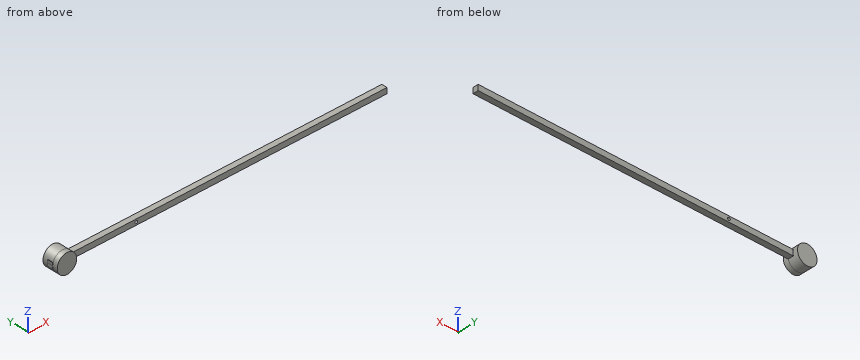
from build123d import *

# Parameters (mm, degrees)
F1_DEPTH      = 10
F3_DEPTH      = 8.75
F3_DEPTH_BACK = 18.75


with BuildPart() as f1:
    # F0 (on Front) → F1 (new body)
    with BuildSketch(Plane.XZ):
        with BuildLine():
            Line((-150, -5), (300, -5))
            Line((300, -5), (300, 5))
            Line((300, 5), (-150, 5))
            ThreePointArc((-150, 5), (-146.464466, 3.535534), (-145, 0))
            ThreePointArc((-145, 0), (-146.464466, -3.535534), (-150, -5))
        make_face()
        with BuildLine():
            Line((-300, -5), (-150, -5))
            ThreePointArc((-150, -5), (-153.535534, -3.535534), (-155, 0))
            Line((-155, 0), (-300, 0))
            Line((-300, 0), (-300, -5))
        make_face()
        with BuildLine():
            Line((-300, 0), (-155, 0))
            ThreePointArc((-155, 0), (-153.535534, 3.535534), (-150, 5))
            Line((-150, 5), (-300, 5))
            Line((-300, 5), (-300, 0))
        make_face()
        with BuildLine():
            ThreePointArc((-155, 0), (-153.535534, -3.535534), (-150, -5))
            ThreePointArc((-150, -5), (-146.464466, -3.535534), (-145, 0))
            ThreePointArc((-145, 0), (-146.464466, 3.535534), (-150, 5))
            ThreePointArc((-150, 5), (-153.535534, 3.535534), (-155, 0))
        make_face()
        with BuildLine():
            ThreePointArc((-147.5, 0), (-150, -2.5), (-152.5, 0))
            ThreePointArc((-152.5, 0), (-150, 2.5), (-147.5, 0))
        make_face(mode=Mode.SUBTRACT)
    extrude(amount=F1_DEPTH)

    # F2 (on face) → F3 (join, two sides)
    with BuildSketch(Plane.XZ.offset(10)) as f3_sk:
        with BuildLine():
            ThreePointArc((-300, 0), (-282.5, -17.5), (-265, 0))
            ThreePointArc((-265, 0), (-282.5, 17.5), (-300, 0))
        make_face()
    extrude(amount=F3_DEPTH)
    extrude(f3_sk.sketch, amount=-F3_DEPTH_BACK)


solid = f1.part
Input: part model. Units: mm. Frame: model coordinates. Coordinates: 2 decimals unless noted, no trailing zeros. Loops run counter-clockwise (first coordinate to the right, second up) from the corner with the lowest first, then second, coordinate; pieces in that order, holes last. Notation, with made-up numbers: (7.25, -31.5) - (63.25, -31.5) arc R12 cw to (63.25, -14.5) - close; hole circle Ø8 at (23, 81). An arc over 180 degrees is marked (long way). Answer in a Markdown table with one row per item. Add a question column.
Item 1: Contact query for flat-ended pins moving along their axis: P1, Ø8, axis at x = 217.5, z = -1.5, coming from the +Y side; P2, Ø6, axis at y = -16, z = 8, coming from the +X side; P3, Ø3, axis at x = -94.5, z = 0, coming from the -Y side. Output: stop coordinate, or through.
Item 2: Line query: line 1 along Z through (x, y) = (-150, -5.75); line 2 along X through (y, z) = (4.5, -0.5); line 3 along Z through (x, y) = (-231, -4.75). Output: solid intervals per line, ascending. Write a range as [from, to].
Item 3: Section query A-A on x = -134.5. Return the cut outline in (y, z), then the cut area to 3 significant figures.
Recorded:
| question | item | result |
|---|---|---|
| 1 | P1 | y = 0 |
| 1 | P2 | x = -265.73 |
| 1 | P3 | y = -10 |
| 2 | line 1 | [-5, -2.5], [2.5, 5] |
| 2 | line 2 | [-299.99, -265.01] |
| 2 | line 3 | [-5, 5] |
| 3 | outline | (-10, -5) - (0, -5) - (0, 5) - (-10, 5) - close |
| 3 | area | 100 mm^2 |
